```python
from build123d import *

# Parameters (mm, degrees)
SKETCH1_R               = 20
BOSS_EXTRUDE1_DEPTH     = 20
SKETCH2_R               = 5
CUT_EXTRUDE1_DEPTH      = 20
SKETCH3_R               = 10
SKETCH3_R_2             = 5
BOSS_EXTRUDE2_DEPTH     = 10
CUT_EXTRUDE2_REACH      = 43.231
CUT_EXTRUDE2_END_RADIUS = 5
SKETCH5_R               = 1


with BuildPart() as part:
    # Sketch1 → Boss-Extrude1 (new body)
    with BuildSketch(Plane.XY):
        Circle(SKETCH1_R)
    extrude(amount=BOSS_EXTRUDE1_DEPTH)

    # Sketch2 → Cut-Extrude1 (cut)
    with BuildSketch(Plane.XY.offset(20)):
        Circle(SKETCH2_R)
    extrude(amount=-CUT_EXTRUDE1_DEPTH, mode=Mode.SUBTRACT)

    # Sketch3 → Boss-Extrude2 (add)
    with BuildSketch(Plane(origin=(0, 0, 0), x_dir=(-1, 0, 0), z_dir=(0, 0, -1))):
        with Locations(Location((0, 0, 0), (0, 0, 180))):
            Circle(SKETCH3_R)
        with Locations(Location((0, 0, 0), (0, 0, 180))):
            Circle(SKETCH3_R_2, mode=Mode.SUBTRACT)
    extrude(amount=BOSS_EXTRUDE2_DEPTH)

    # Cut-Extrude2: up to this cylinder (the profile starts outside it)
    cut_extrude2_end = Plane(origin=(0, 0, -5), z_dir=(0, 0, 1)) * Cylinder(CUT_EXTRUDE2_END_RADIUS, 97.462, mode=Mode.PRIVATE)
    # Sketch5 → Cut-Extrude2 (cut, up to the surface)
    with BuildSketch(Plane(origin=(10, 0, 0), x_dir=(0, 0, -1), z_dir=(1, 0, 0)), mode=Mode.PRIVATE) as cut_extrude2_sk1:
        with Locations((5, 0)):
            Circle(SKETCH5_R)
    cut_extrude2_tool1 = extrude(cut_extrude2_sk1.sketch, amount=-CUT_EXTRUDE2_REACH, mode=Mode.PRIVATE) - cut_extrude2_end
    add(cut_extrude2_tool1.solids().sort_by_distance((10, 0, -5))[0], mode=Mode.SUBTRACT)


solid = part.part
```
Model file for the job. Use its own axes, mm. A direction names the side the tool comes from. Coordinates: 2 decimals unless noted, no trailing zeros. Write each loop counter-clockwise with the first axis right and the second up, starting at its lowest first coordinate (ties: lowest second). Pieces come first, ordered by that corner, then holes. Notation, with made-up numbers: (1.5, 22.25) - (15.5, 22.25) arc R18 ccw to (15.5, 36.25) - close; hole circle Ø10 at (-18, 55.5). An arc over 180 degrees is marked (long way). Use a Markdown table: item, result. Add a question column.
Item 1: Band-saw the part on C-C, the plane z = 13.5. Write the cut outline in (x, y), and give its area (3 significant figures).
Item 2: 3-axis set-ups, long thin cutter, end or side, ignore diameter. For faces 1 (the face through (2, -5, -10)), 2 (the face through (-5, 9, 0)): which of +Z, -Z, +X, -X, +Y, -Y reach the whole face in a straight line?
Item 3: Band-saw the part on B-B, the plane y = 0. Write the cut outline in (x, z), and give its area (3 significant figures).
Item 4: Drop flat-ended pins along their axis: pin 1 (4 mm diameter, centred on y = -12.5, z = -0.5, fed in from +X); pin 2 (1 mm diameter, centred on y = -4.5, z = 14, fed in from +X); pin 3 (1.5 mm diameter, centred on x = -11, z = 0.5, fed in from -Y). Give the stop position or say it passes through.
Item 5: Drill centre lines: line 1 along Y through (x, z) = (0, -3.75); line 2 along Z through (x, y) = (8.5, 8.5). Where is each one in solid material? Low to high.
Item 6: Two-plate mould, pull along Y, no slides. Class faces 3 (the face through (7.5, -0.6, -4.2)), 4 (the face through (-4.336, -19.524, 9.86)), 5 (the face through (4, -4, 20)): pulls with the +Y half, pulls with the -Y half, needs draft (parallel to the pull), parting line crosses it, or undercut.
Item 7: Band-saw the part on A-A, the plane x = 0. Write the cut outline in (y, z), and give its area (3 significant figures).
Item 8: Band-saw the part on D-D, the plane x = -6.5. Write the cut outline in (y, z).
A:
| question | item | result |
|---|---|---|
| 1 | outline | circle Ø40 at (0, 0); hole circle Ø10 at (0, 0) |
| 1 | area | 1,180 mm² |
| 2 | face 1 | -Z, +X, -X, +Y, -Y |
| 2 | face 2 | -Z |
| 3 | outline | (-20, 0) - (-10, 0) - (-10, -10) - (-5, -10) - (-5, 20) - (-20, 20) - close; (5, -10) - (10, -10) - (10, -6) - (5, -6) - close; (5, -4) - (10, -4) - (10, 0) - (20, 0) - (20, 20) - (5, 20) - close |
| 3 | area | 690 mm² |
| 4 | pin 1 | stops at x = 16.98 |
| 4 | pin 2 | stops at x = 19.6 |
| 4 | pin 3 | stops at y = -17.17 |
| 5 | line 1 | y = -10 to -5, 5 to 10 |
| 5 | line 2 | z = 0 to 20 |
| 6 | face 3 | undercut |
| 6 | face 4 | parting line crosses it |
| 6 | face 5 | needs draft |
| 7 | outline | (-20, 0) - (-10, 0) - (-10, -10) - (-5, -10) - (-5, 20) - (-20, 20) - close; (5, -10) - (10, -10) - (10, 0) - (20, 0) - (20, 20) - (5, 20) - close |
| 7 | area | 700 mm² |
| 8 | outline | (-18.91, 0) - (-7.6, 0) - (-7.6, -10) - (7.6, -10) - (7.6, 0) - (18.91, 0) - (18.91, 20) - (-18.91, 20) - close |
